Check sheet for the modelled part. Datum: model origin and axes. Units: mm. Face numbers are marked on the shaded views. A direction names the side the tool comes from. Coordinates: 2 decimals unless noted, no trailing zeros. Loops run counter-clockwise (first coordinate to the right, second up) from the corner with the lowest first, then second, coordinate; pieces in that order, holes last. Notation, with made-up numbers: (36, 11.5) - (64, 11.5) arc R32 cw to (64, 40.5) - close; hole circle Ø6 at (-15, 53.5). An arc over 180 degrees is marked (long way). Use a Markdown table: item, result. Add a question column.
1) Tool access check on the marked faces 5, 6 and 7. Record the directions out of +Z, -Z, +X, -X, +Y, -Y that give a thin tool (end or side, any length) a straight path to the whole face; none if there is none.
2) Sectioned sample at C-C, the plane y = -19. Enter the section's corners in (x, z), then the cut area to 3 significant figures.
3) Sectioned sample at B-B, the plane x = 2.25. State how many separate pieces and enclosed holes the cut face has, then the cut area to 3 significant figures.
4) Draft check along Y on the marked faces 1, 2, 3 and 4. Enter one of: pulls with the +Y half, pulls with the -Y half, needs draft (parallel to the pull), parting line crosses it, or undercut.
5) Go/stop test with flat-tipped pins: P1, Ø8, axis at x = 7.5, y = 9, coming from the -Z side; P2, Ø13, axis at x = -1, z = -0.5, coming from the -Y side; P3, Ø0.7, axis at x = 9.5, y = -3.5, coming from the -Z side; P4, Ø2, axis at x = 9, z = 19, coming from the +Y side. Record where each tip stops, or that it passes through.
6) Sectioned sample at A-A, the plane y = 5.5. Enter the section's corners in (x, z).
7) Thickness scan on line 1 (Y direction, x = 0, z = 18); line 2 (Y direction, x = 0, z = 25.5); line 3 (Z direction, x = 0, y = -6.75). Record the ranges inside material, lowest first.
from build123d import *

# Parameters (mm, degrees)
CROQUIS2_R                 = 12.488984619
SALIENTE_EXTRUIR1_DEPTH    = 28
CROQUIS3_R                 = 9
CORTAR_EXTRUIR1_DEPTH      = 19.788850508
CORTAR_EXTRUIR1_DEPTH_BACK = 31.711149692
CROQUIS4_R                 = 13.25
SALIENTE_EXTRUIR2_DEPTH    = 6.5
CORTAR_EXTRUIR2_REACH      = 44.659
CROQUIS5_R                 = 9.25


with BuildPart() as part:
    # Croquis1 → Revolución1 (revolve)
    with BuildSketch(Plane.XY):
        Polygon((11.12, 18.788850408), (13.2, 18.788850408), (13.2, 13.288850408), (12.5, 13.288850408), (12.5, -25.211149592), (14.659269355, -25.211149592), (14.659269355, -30.711149592), (11.12, -30.711149592), (9.525, -16.252125457), (10.31589022, -16.252125457), (10.31589022, 7.254829614), (9.525, 7.254829614), align=None)
    revolve(axis=Axis((0, 29.936319964, 0), (0, -1, 0)))

    # Croquis2 → Saliente-Extruir1 (add)
    with BuildSketch(Plane.XY):
        with Locations((0, -4.438102688)):
            Circle(CROQUIS2_R)
    extrude(amount=SALIENTE_EXTRUIR1_DEPTH)

    # Croquis3 → Cortar-Extruir1 (cut, two sides)
    with BuildSketch(Plane(origin=(0, 0, 0), x_dir=(1, 0, 0), z_dir=(0, 1, 0))) as cortar_extruir1_sk:
        Circle(CROQUIS3_R)
    extrude(amount=CORTAR_EXTRUIR1_DEPTH, mode=Mode.SUBTRACT)
    extrude(cortar_extruir1_sk.sketch, amount=-CORTAR_EXTRUIR1_DEPTH_BACK, mode=Mode.SUBTRACT)

    # Croquis4 → Saliente-Extruir2 (add)
    with BuildSketch(Plane.XY.offset(28)):
        with Locations((0, -4.438102688)):
            Circle(CROQUIS4_R)
    extrude(amount=-SALIENTE_EXTRUIR2_DEPTH)

    # Croquis5 → Cortar-Extruir2 (cut, up to next)
    with BuildSketch(Plane.XY.offset(28), mode=Mode.PRIVATE) as cortar_extruir2_sk1:
        with Locations((0, -4.438102688)):
            Circle(CROQUIS5_R)
    cortar_extruir2_tool1 = extrude(cortar_extruir2_sk1.sketch, amount=-CORTAR_EXTRUIR2_REACH, mode=Mode.PRIVATE) & part.part
    add(cortar_extruir2_tool1.solids().sort_by_distance((0, -4.438103, 28))[0], mode=Mode.SUBTRACT)


solid = part.part
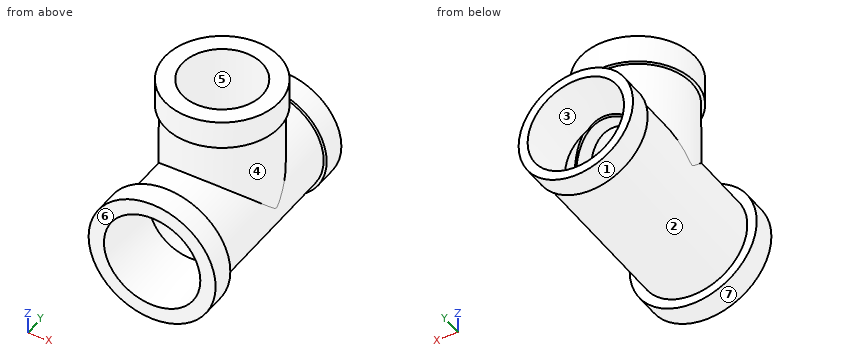
Solved:
| question | item | result |
|---|---|---|
| 1 | face 5 | +Z |
| 1 | face 6 | +Z, -Z, +X, -X, -Y |
| 1 | face 7 | -Y |
| 2 | outline | circle Ø25 at (0, 0); hole circle Ø19.66 at (0, 0) |
| 2 | area | 187 mm2 |
| 3 | separate pieces | 3 |
| 3 | enclosed holes | 0 |
| 3 | area | 334 mm2 |
| 4 | face 1 | needs draft |
| 4 | face 2 | undercut |
| 4 | face 3 | pulls with the +Y half |
| 4 | face 4 | undercut |
| 5 | P1 | stops at z = -12 |
| 5 | P2 | passes through |
| 5 | P3 | stops at z = -8.52 |
| 5 | P4 | stops at y = 5.15 |
| 6 | outline | (-8.76, 21.5) - (-7.56, 21.5) - (-7.56, 9.95) arc R12.5 ccw (long way) to (7.56, 9.95) - (7.56, 21.5) - (8.76, 21.5) - (8.76, 28) - (-8.76, 28) - close; hole (-7.56, 4.88) - (-7.56, 7.01) arc R10.32 ccw (long way) to (7.56, 7.01) - (7.56, 4.88) arc R9 ccw to start |
| 7 | line 1 | y = -16.93 to -13.69, 4.81 to 8.05 |
| 7 | line 2 | y = -17.69 to -13.69, 4.81 to 8.81 |
| 7 | line 3 | z = -12.5 to -10.32 |
